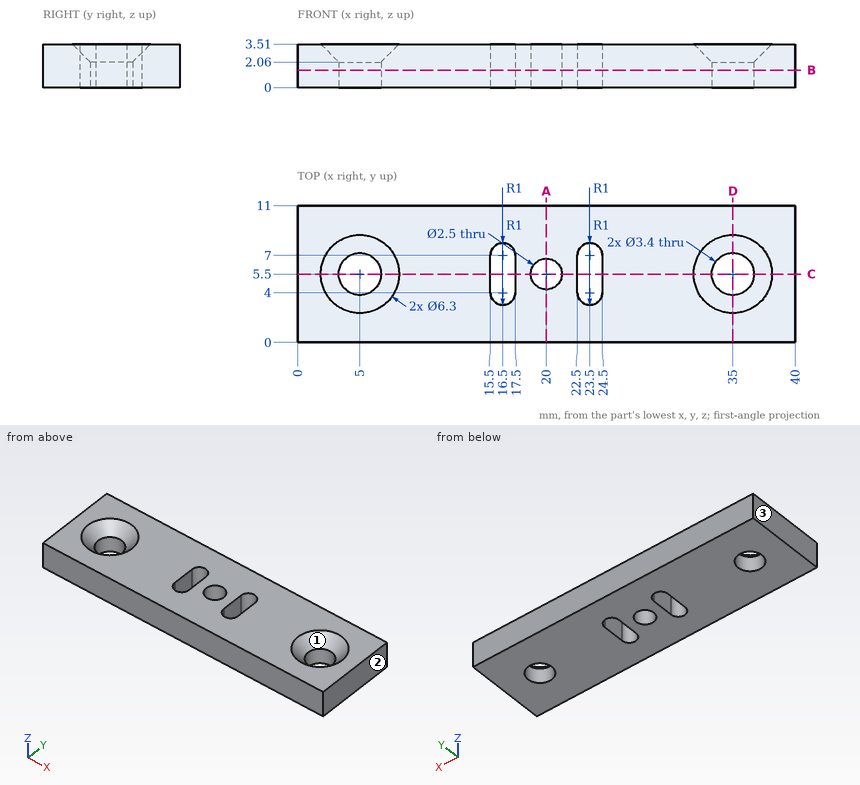
Verification items for this drawing (mm, ordinates from the low corner). Give positions to 0.01 mm unless a question says otherwise; leave off trailing zeros. Write each loop counter-clockwise with the first axis right and the second up, starting at its lowest first coordinate (ties: lowest second). Pieces come first, ordered by that corner, then holes. Notation, with made-up numbers: (43.5, 20.25) - (69.5, 20.25) arc R10 ccw to (69.5, 29.25) - close; hole circle Ø3 at (41, 42.25). An arc over 180 degrees is marked (long way). Answer as a JSON object with one key per item and string values. Group by question number.
1) Release check for a two-part mould opening along X. For the marked faces 1, 2 and 3 record: pulls with the +X half, pulls with the -X half, needs draft (parallel to the pull), parting line crosses it, or undercut.
2) Sectioned sample at D-D (x = 35). Record the cut outline in (y, z).
3) Thickness scan on probe 1 along Y at (x, z) = (20, 0.85); probe 2 along X at (y, z) = (6, 2); probe 3 along X at (y, z) = (4, 3.1). Record the ranges inside material, lowest first. Write a range as from..to.
4) Sectioned sample at C-C (y = 5.5). Record the cut outline in (x, z).
5) Sectioned sample at A-A (x = 20). Record the cut outline in (y, z).
6) Depth check by flat-ended pin: P1, Ø5, axis at x = 14.5, y = 9, coming from the -Z side; P2, Ø2.5, axis at x = 5, y = 5.5, coming from the +Z side. Enter the tip coordinate at first touch or a pass-through.
7) Sectioned sample at B-B (z = 1.4). Record the cut outline in (x, y).
Geometry results:
{
 "1": {"face 1": "undercut", "face 2": "pulls with the +X half", "face 3": "pulls with the -X half"},
 "2": {"outline": "(0, 0) - (3.8, 0) - (3.8, 2.06) - (2.35, 3.51) - (0, 3.51) - close; (7.2, 0) - (11, 0) - (11, 3.51) - (8.65, 3.51) - (7.2, 2.06) - close"},
 "3": {"probe 1": "y = 0..4.25, 6.75..11", "probe 2": "x = 0..3.38, 6.62..15.5, 17.5..18.85, 21.15..22.5, 24.5..33.38, 36.62..40", "probe 3": "x = 0..2.71, 7.29..15.5, 17.5..22.5, 24.5..32.71, 37.29..40"},
 "4": {"outline": "(0, 0) - (3.3, 0) - (3.3, 2.06) - (1.85, 3.51) - (0, 3.51) - close; (6.7, 0) - (15.5, 0) - (15.5, 3.51) - (8.15, 3.51) - (6.7, 2.06) - close; (17.5, 0) - (18.75, 0) - (18.75, 3.51) - (17.5, 3.51) - close; (21.25, 0) - (22.5, 0) - (22.5, 3.51) - (21.25, 3.51) - close; (24.5, 0) - (33.3, 0) - (33.3, 2.06) - (31.85, 3.51) - (24.5, 3.51) - close; (36.7, 0) - (40, 0) - (40, 3.51) - (38.15, 3.51) - (36.7, 2.06) - close"},
 "5": {"outline": "(0, 0) - (4.25, 0) - (4.25, 3.51) - (0, 3.51) - close; (6.75, 0) - (11, 0) - (11, 3.51) - (6.75, 3.51) - close"},
 "6": {"P1": "stops at z = 0", "P2": "passes through"},
 "7": {"outline": "(0, 0) - (40, 0) - (40, 11) - (0, 11) - close; hole circle Ø3.4 at (5, 5.5); hole (15.5, 4) arc R1 ccw to (17.5, 4) - (17.5, 7) arc R1 ccw to (15.5, 7) - close; hole circle Ø2.5 at (20, 5.5); hole (22.5, 4) arc R1 ccw to (24.5, 4) - (24.5, 7) arc R1 ccw to (22.5, 7) - close; hole circle Ø3.4 at (35, 5.5)"}
}
